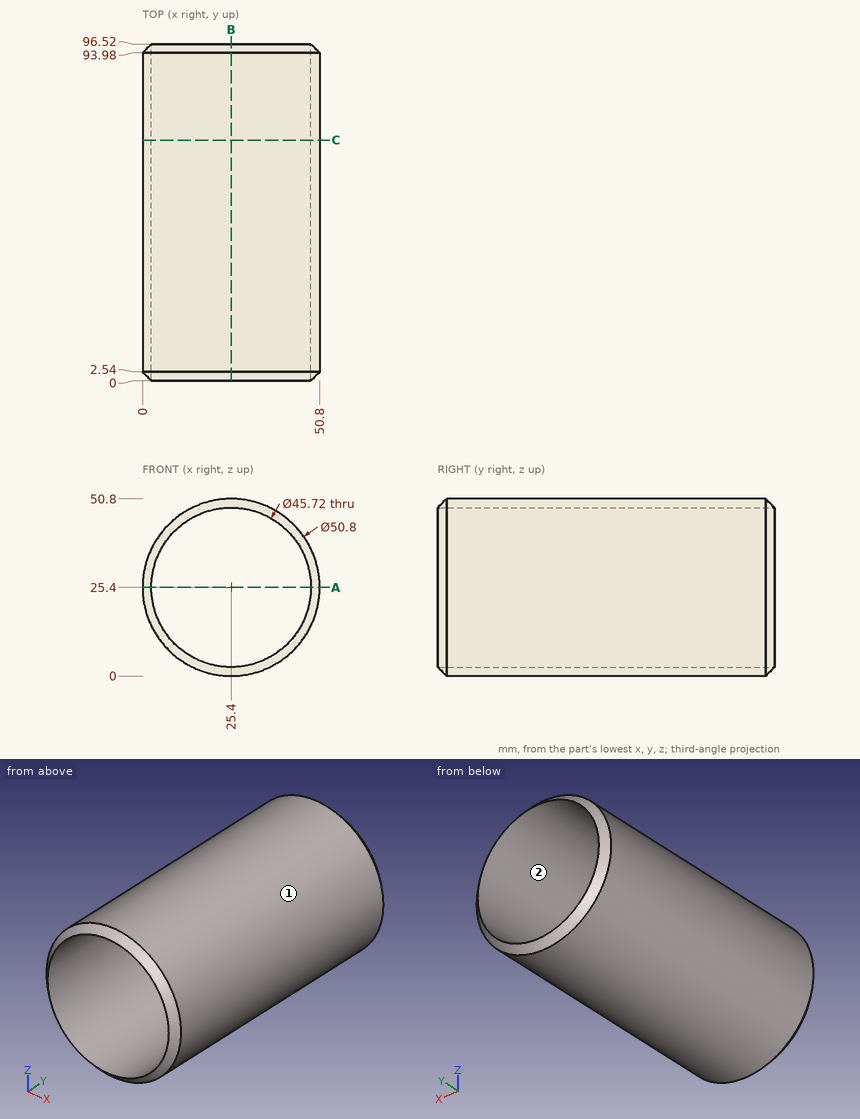
Answer from the drawing. Dimensions are ordinates in mm from the lowest x, y and z of the part. Round coordinates to 2 decimals unless told otherwise and drop trailing zeros. Write each loop counter-clockwise with the first axis right and the second up, starting at its lowest first coordinate (ties: lowest second). Pieces come first, ordered by that corner, then holes. Notation, with made-up numbers: (-22.5, 19.25) - (-11.5, 19.25) arc R22 cw to (-11.5, 28.25) - close; hole circle Ø11 at (-22, -18). An arc over 180 degrees is marked (long way). One line per item, written item: value.
Q1. Straight lines are drawn through the part: line 1 (Z direction, x = 25, y = 76); line 2 (Z direction, x = 24.5, y = 50); line 3 (X direction, y = 50, z = 14). For each, find the intervals that lie inside material, in ascending order. Write a range as from..to.
The answers:
line 1: z = 0..2.54, 48.26..50.8
line 2: z = 0.02..2.56, 48.24..50.78
line 3: x = 2.7..5.59, 45.21..48.1
Q2. For a pull along Z with two mould halves and no side action, classify the marked faces 1 and 2 as pulls with the +Z half, pulls with the -Z half, needs draft (parallel to the pull), parting line crosses it, or undercut.
The answers:
face 1: parting line crosses it
face 2: undercut
Q3. Find section C-C (y = 69). Determine the outline of the cut face in (x, z), and give its area (3 significant figures).
The answers:
outline: circle Ø50.8 at (25.4, 25.4); hole circle Ø45.72 at (25.4, 25.4)
area: 385 mm2
Q4. Find section B-B (x = 25.4). Determine the outline of the cut face in (y, z).
The answers:
outline: (0, 2.54) - (2.54, 0) - (93.98, 0) - (96.52, 2.54) - close; (0, 48.26) - (96.52, 48.26) - (93.98, 50.8) - (2.54, 50.8) - close
Q5. Find section A-A (z = 25.4). Determine the outline of the cut face in (x, y).
The answers:
outline: (0, 2.54) - (2.54, 0) - (2.54, 96.52) - (0, 93.98) - close; (48.26, 0) - (50.8, 2.54) - (50.8, 93.98) - (48.26, 96.52) - close
Q6. Each of these flat-tipped pins is pushed along its axis until it touches: P1, Ø6, axis at y = 15, z = 17.5, coming from the +X side; P2, Ø12, axis at y = 85, z = 8.5, coming from the +X side; P3, Ø12, axis at y = 79, z = 17.5, coming from the +X side; P4, Ø12, axis at x = 15, z = 36, coming from the +Y side. Where does it stop, or does it pass through?
The answers:
P1: stops at x = 50.32
P2: stops at x = 48.34
P3: stops at x = 50.73
P4: passes through
